Source: three-view drawing plus pictorial views. Frame: mm from the lowest corner of the part. Round coordinates to 2 decimals unless told otherwise and drop trailing zeros. Loops run counter-clockwise (first coordinate to the right, second up) from the corner with the lowest first, then second, coordinate; pieces in that order, holes last. Notation, with made-up numbers: M 64.5,29 L 115.5,29 A26 ccw 115.5,59 Z; hole C 7.25,80 d1. An arc over 180 degrees is marked long. Answer as a JSON object with one key per item and string values.
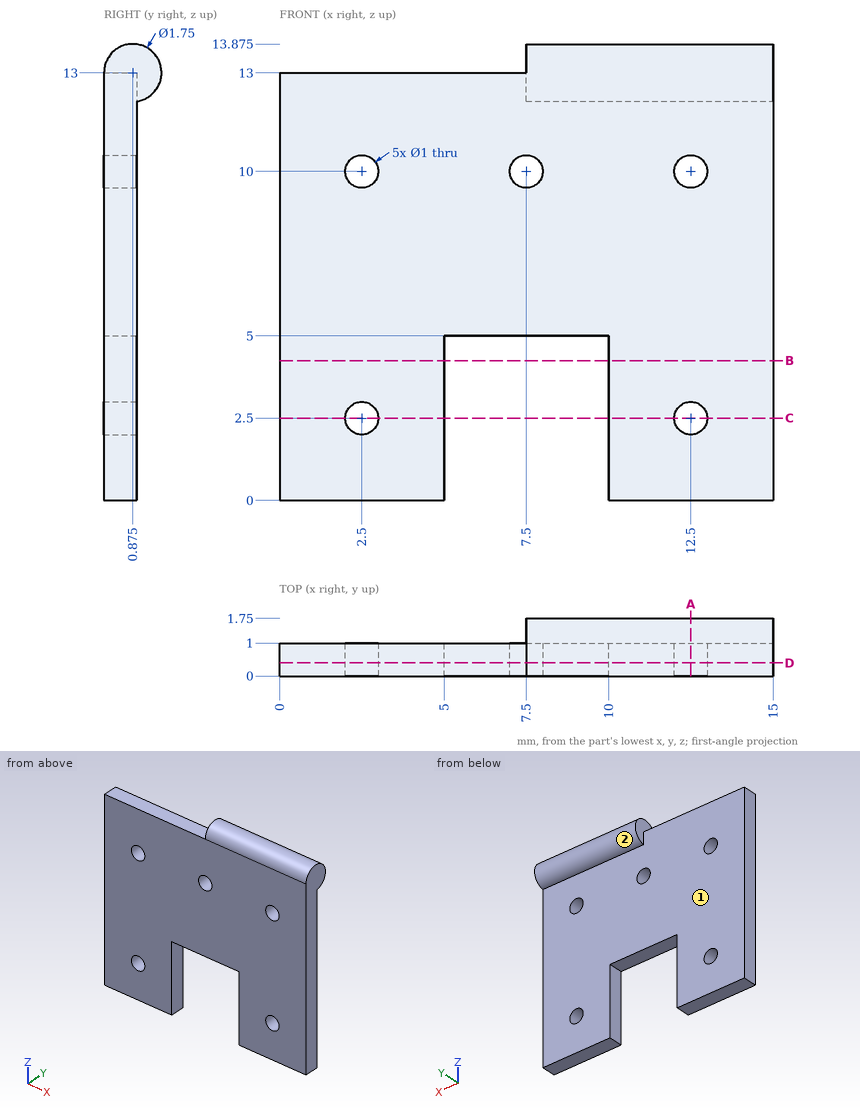
1) First-contact query: pin 1 (4 mm diameter, centred on x = 8.5, z = 2, fed in from +Y). Flat tip, straight axial feed; report the tip coordinate or a pass-through.
Geometry results:
{"pin 1": "y = 1"}
2) Cut plane D-D on y = 0.4. Return the cut outline in (x, z), and give its area (3 significant figures).
Geometry results:
{"outline": "M 0,0 L 5,0 L 5,5 L 10,5 L 10,0 L 15,0 L 15,13.73 L 7.5,13.73 L 7.5,13 L 0,13 Z; hole C 2.5,2.5 d1; hole C 2.5,10 d1; hole C 7.5,10 d1; hole C 12.5,2.5 d1; hole C 12.5,10 d1", "area": "172 mm2"}
3) Cut plane B-B on z = 4.25. Return the cut outline in (x, y), and give its area (3 significant figures).
Geometry results:
{"outline": "M 0,0 L 5,0 L 5,1 L 0,1 Z; M 10,0 L 15,0 L 15,1 L 10,1 Z", "area": "10.0 mm2"}
4) Cut plane A-A on x = 12.5. Return the cut outline in (y, z) (3 decimals).
Geometry results:
{"outline": "M 0,0 L 1,0 L 1,2 L 0,2 Z; M 0,3 L 1,3 L 1,9.5 L 0,9.5 Z; M 0,10.5 L 1,10.5 L 1,12.134 A0.875 ccw long 0,13 Z"}
5) Cut plane C-C on z = 2.5. Return the cut outline in (x, y).
Geometry results:
{"outline": "M 0,0 L 2,0 L 2,1 L 0,1 Z; M 3,0 L 5,0 L 5,1 L 3,1 Z; M 10,0 L 12,0 L 12,1 L 10,1 Z; M 13,0 L 15,0 L 15,1 L 13,1 Z"}
6) Line query: probe 1 along X at (y, z) = (0.45, 2.5); probe 2 along X at (y, z) = (0.35, 10); probe 3 along Z at (x, y) = (2.5, 0.65). Output: solid intervals per line, ascending.
Geometry results:
{"probe 1": "0 to 2, 3 to 5, 10 to 12, 13 to 15", "probe 2": "0 to 2, 3 to 7, 8 to 12, 13 to 15", "probe 3": "0 to 2, 3 to 9.5, 10.5 to 13"}
7) Pull-direction query (Z, two-part tool) for the marked faces 1 and 2; classes: +Z half, -Z half, draft (parallel to the pull), parting line (faces both ways), or undercut.
Geometry results:
{"face 1": "draft", "face 2": "parting line"}
